Read the model definition and answer for the solid it produces. Units are mm, in the model's axes. A direction names the side the tool comes from. Coordinates: 2 decimals unless noted, no trailing zeros. Loops run counter-clockwise (first coordinate to the right, second up) from the corner with the lowest first, then second, coordinate; pieces in that order, holes last. Notation, with made-up numbers: (-18.75, -9) -> (-3.75, -9) arc R17 ccw to (-3.75, -1) -> close; hole circle Ø3 at (-10, 33). An arc over 180 degrees is marked (long way). Answer as CSV lines item,"result".
```python
from build123d import *

# Parameters (mm, degrees)
F0_W     = 92
F0_H     = 230
F1_DEPTH = 4
F3_D     = 9
F4_D     = 12
F6_DEPTH = 4


with BuildPart() as f1:
    # F0 (on Front) → F1 (new body)
    with BuildSketch(Plane.XZ):
        with Locations((46, 115)):
            Rectangle(F0_W, F0_H)
    extrude(amount=F1_DEPTH)

    # F3 (through all)
    with Locations(Plane.XZ.offset(4)):
        with Locations((16, 8), (76, 8)):
            Hole(F3_D / 2)

    # F4 (through all)
    with Locations(Plane.XZ.offset(4)):
        with Locations((46, 220)):
            Hole(F4_D / 2)

    # F5 (on face) → F6 (cut, through all)
    with BuildSketch(Plane.XZ.offset(4)):
        with BuildLine():
            ThreePointArc((41, 100), (46, 95), (51, 100))
            Line((51, 100), (51, 196))
            ThreePointArc((51, 196), (46, 201), (41, 196))
            Line((41, 196), (41, 100))
        make_face()
    extrude(amount=-F6_DEPTH, mode=Mode.SUBTRACT)


solid = f1.part
```
Q1. A cutting plane is placed at A-A, the plane x = 46. Write down the section's boundary in (y, z).
Results:
outline,"(-4, 0) -> (0, 0) -> (0, 95) -> (-4, 95) -> close; (-4, 201) -> (0, 201) -> (0, 214) -> (-4, 214) -> close; (-4, 226) -> (0, 226) -> (0, 230) -> (-4, 230) -> close"
Q2. A cutting plane is placed at B-B, the plane z = 186.5. Write down the section's boundary in (x, y), and give its area (3 significant figures).
Results:
outline,"(0, -4) -> (41, -4) -> (41, 0) -> (0, 0) -> close; (51, -4) -> (92, -4) -> (92, 0) -> (51, 0) -> close"
area,"328 mm²"
Q3. A cutting plane is placed at C-C, the plane x = 16. Write down the section's boundary in (y, z), and give its area (3 significant figures).
Results:
outline,"(-4, 0) -> (0, 0) -> (0, 3.5) -> (-4, 3.5) -> close; (-4, 12.5) -> (0, 12.5) -> (0, 230) -> (-4, 230) -> close"
area,"884 mm²"
Q4. A cutting plane is placed at D-D, the plane z = 8. Write down the section's boundary in (x, y).
Results:
outline,"(0, -4) -> (11.5, -4) -> (11.5, 0) -> (0, 0) -> close; (20.5, -4) -> (71.5, -4) -> (71.5, 0) -> (20.5, 0) -> close; (80.5, -4) -> (92, -4) -> (92, 0) -> (80.5, 0) -> close"
Q5. For faces 4 (the face through (45, -2, 0)), 5 (the face through (46, -2, 95)), determine the directions among +Z, -Z, +X, -X, +Y, -Y from which every point of the face is accessible in a straight line to the end or side of a thin tool.
Results:
face 4,"-Z, +X, -X, +Y, -Y"
face 5,"+Y, -Y"
Q6. Find the intervals of material crossed by probe 1 along Z at (x, y) = (46, -2.25); probe 2 along Z at (x, y) = (16, -2); probe 3 along X at (y, z) = (-2.4, 101), in increasing order. Write a range as [from, to].
Results:
probe 1,"z = [0, 95], [201, 214], [226, 230]"
probe 2,"z = [0, 3.5], [12.5, 230]"
probe 3,"x = [0, 41], [51, 92]"
Q7. For a pull along Z with two mould halves and no side action, classify faces 1 (the face through (50.76, -1.97, 216.35)), 2 (the face through (35, -4, 117)), 3 (the face through (45, -2, 230)) as pulls with the +Z half, pulls with the -Z half, needs draft (parallel to the pull), parting line crosses it, or undercut.
Results:
face 1,"undercut"
face 2,"needs draft"
face 3,"pulls with the +Z half"
